For this review, take the finished solid that the model builds, in its own axes (mm). A direction names the side the tool comes from. Round coordinates to 2 decimals unless told otherwise and drop trailing zeros. Loops run counter-clockwise (first coordinate to the right, second up) from the corner with the lowest first, then second, coordinate; pieces in that order, holes last.
1) Tool access review of faces 4 (the flat face through (73, 10, -17)), 5 (the flat face through (17, 0, 75)), 6 (the flat face through (73, -152.4, -17)): name each direction out of +Z, -Z, +X, -X, +Y, -Y from which nothing blocks a thin tool from reaching the whole face with its end or side.
2) Take a section at A-A (y = -35). State the section outline as (x, z) points, then the cut area to 3 significant figures.
3) Mouldability with a two-part tool opening along X and no side actions: class faces 1 (the flat face through (7.34, 370, -7.35)), 2 (the cylindrical face through (46.367, -77.267, 60.47)), 3 (the cylindrical face through (22.288, -72.337, 70.774)) as pulls with the +X half, pulls with the -X half, needs draft (parallel to the pull), parting line crosses it, or undercut.
4) Wall thickness on L1, parallel to X at y = -91.5, z = 0; L2, parallel to X at y = 211, z = 36; L3, parallel to Z at x = -58, y = -98.5: over which ranges is each line inside the solid? List them lowest first.
5) Insertion check: pin 1 (12 mm diameter, centred on y = 269.5, z = 25, fed in from -X); pin 2 (6 mm diameter, centred on y = 186, z = -35, fed in from +X); pin 3 (8 mm diameter, centred on y = -99.5, z = -34.5, fed in from -X). Each pin has a flat end and moves straight along its axis. Give the tip position at first contact, or say it passes through.
```python
from build123d import *

# Parameters (mm, degrees)
BOSS_EXTRUDE1_DEPTH      = 10
BOSS_EXTRUDE1_DEPTH_BACK = 152.4
SKETCH2_R                = 76.2
SKETCH2_R_2              = 74.2
SKETCH6_R                = 45.027407712
CUT_EXTRUDE1_DEPTH       = 40


with BuildPart() as part:
    # Sketch1 → Revolve3 (revolve)
    with BuildSketch(Plane.XY):
        with BuildLine():
            Line((0, 400), (0, 401.853426775))
            ThreePointArc((0, 401.853426775), (58.468341276, 204.695759977), (78.2, 0))
            Line((78.2, 0), (76.2, 0))
            ThreePointArc((76.2, 0), (56.977268898, 201.872568324), (0, 396.489212171))
            Line((0, 396.489212171), (0, 400))
        make_face()
    revolve(axis=Axis((0, 400, 0), (0, 1, 0)))

    # Sketch2 → Boss-Extrude1 (add, two sides: drawn at the far end of the back side and taken through both)
    with BuildSketch(Plane(origin=(0, 0, 0), x_dir=(1, 0, 0), z_dir=(0, 1, 0)).offset(-BOSS_EXTRUDE1_DEPTH_BACK)):
        with Locations(Location((0, 0, 0), (0, 0, 90))):
            Circle(SKETCH2_R)
        with Locations(Location((0, 0, 0), (0, 0, 270))):
            Circle(SKETCH2_R_2, mode=Mode.SUBTRACT)
    extrude(amount=BOSS_EXTRUDE1_DEPTH + BOSS_EXTRUDE1_DEPTH_BACK)

    # Sketch6 → Cut-Extrude1 (cut)
    with BuildSketch(Plane(origin=(0, 370, 0), x_dir=(-1, 0, 0), z_dir=(0, -1, 0))):
        Circle(SKETCH6_R)
    extrude(amount=-CUT_EXTRUDE1_DEPTH, mode=Mode.SUBTRACT)


solid = part.part
```
Response:
1. face 4: none
1. face 5: -Y
1. face 6: +Z, -Z, +X, -X, -Y
2. outline: circle Ø152.4 at (0, 0); hole circle Ø148.4 at (0, 0)
2. area: 945 mm2
3. face 1: needs draft
3. face 2: parting line crosses it
3. face 3: undercut
4. L1: x = -76.2 to -74.2, 74.2 to 76.2
4. L2: x = -44.48 to -41.82, 41.82 to 44.48
4. L3: z = -49.42 to -46.28, 46.28 to 49.42
5. pin 1: stops at x = -39.89
5. pin 2: stops at x = 53.13
5. pin 3: stops at x = -69.83
